For this review, take the finished solid that the model builds, in its own axes (mm). A direction names the side the tool comes from. Give positions to 0.01 mm unless a question says otherwise; leave off trailing zeros. Order: outer loops, then holes, each group sorted by start corner. A loop starts at its lowest first (then second) coordinate and runs counter-clockwise, first axis right, second up. Notation, with made-up numbers: (8, 13) - (42, 13) arc R19 ccw to (42, 37) - close; hole circle Ø9 at (14, 84.5). An arc over 180 degrees is marked (long way). Answer as a JSON object with one key per item and string values. Group by question number.
from build123d import *

# Parameters (mm, degrees)
F0_R     = 6.35
F1_DEPTH = 127
F3_DEPTH = 6.35


with BuildPart() as f1:
    # F0 (on Right) → F1 (new body)
    with BuildSketch(Plane.YZ):
        Circle(F0_R)
    extrude(amount=F1_DEPTH)

    # F2 (on face) → F3 (join)
    with BuildSketch(Plane.YZ.offset(127)):
        Polygon((5.499261, 9.525), (-5.499261, 9.525), (-10.998523, 0), (-5.499261, -9.525), (5.499261, -9.525), (10.998523, 0), align=None)
    extrude(amount=F3_DEPTH)


solid = f1.part
1) For faces 1 (the face through (130.131, 8.287, 4.696)), 2 (the face through (127, -0.2, 6.5)), list the 3-axis set-ups (+Z, -Z, +X, -X, +Y, -Y) from which the entire face can be reached by the end or side of a thin tool; tool diameter is ignored.
2) Consider section C-C (x = 91). Give the boundary of the cut face in (y, z), plus the area to 3 significant figures.
3) Consider section B-B (z = 4.5). Give the boundary of the cut face in (x, y), plus the area to 3 significant figures.
4) For line 1 (X direction, y = -6.5, z = -5.5); line 2 (Y direction, x = 16, z = 1.5); line 3 (Z direction, x = 77, y = 2.75), list the stretches that pass through material, from the lowest coordinate up.
5) Consider section A-A (y = 0). Give the boundary of the cut face in (x, z) (3 decimals).
6) For pin 1 (4 mm diameter, centred on x = 81.5, y = 3.5, fed in from +Z); pin 2 (4 mm diameter, centred on x = 69, y = 1.5, fed in from -Z); pin 3 (1.5 mm diameter, centred on x = 77.5, z = -6, fed in from -Y); pin 4 (8 mm diameter, centred on y = 6, z = -3.5, fed in from -X), all flat-tipped, find the tip position at first contact; note any pin that passes through.
Result set:
{
 "1": {"face 1": "+Z, +X, -X, +Y", "face 2": "-X"},
 "2": {"outline": "circle Ø12.7 at (0, 0)", "area": "127 mm2"},
 "3": {"outline": "(0, -4.48) - (127, -4.48) - (127, -8.4) - (133.35, -8.4) - (133.35, 8.4) - (127, 8.4) - (127, 4.48) - (0, 4.48) - close", "area": "1,240 mm2"},
 "4": {"line 1": "x = 127 to 133.35", "line 2": "y = -6.17 to 6.17", "line 3": "z = -5.72 to 5.72"},
 "5": {"outline": "(0, -6.35) - (127, -6.35) - (127, -9.525) - (133.35, -9.525) - (133.35, 9.525) - (127, 9.525) - (127, 6.35) - (0, 6.35) - close"},
 "6": {"pin 1": "stops at z = 6.17", "pin 2": "stops at z = -6.35", "pin 3": "stops at y = -3.57", "pin 4": "stops at x = 0"}
}
